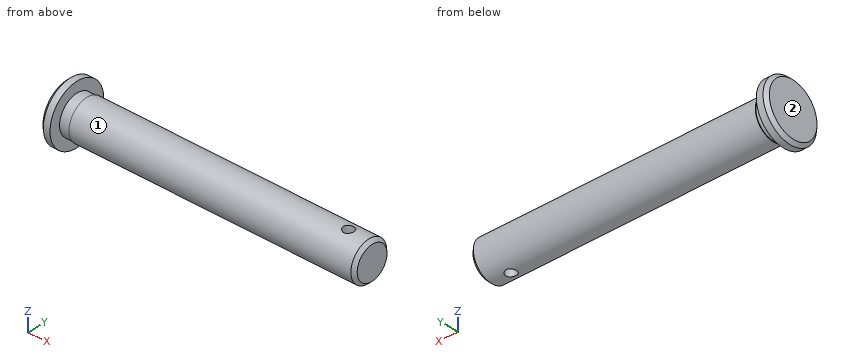
```python
from build123d import *

# Parameters (mm, degrees)
SKETCH2_R          = 0.8
CUT_EXTRUDE1_DEPTH = 46.15517689
CHAMFER1_SIZE      = 0.5


with BuildPart() as part:
    # Sketch1 → Revolve1 (revolve)
    with BuildSketch(Plane.XY, mode=Mode.PRIVATE) as revolve1_sk:
        Polygon((-1.5, 0), (-1.5, 4.5), (0, 4.5), (0, 2.9), (1.5, 2.9), (1.5, 3), (44.3, 3), (44.3, 0), align=None)
    revolve(revolve1_sk.sketch.rotate(Axis((0, 0, 0), (1, 0, 0)), 90), axis=Axis((0, 0, 0), (1, 0, 0)))

    # Sketch2 → Cut-Extrude1 (cut, through all)
    with BuildSketch(Plane.XY.offset(3)):
        with Locations((40.8, 0)):
            Circle(SKETCH2_R)
    extrude(amount=-CUT_EXTRUDE1_DEPTH, mode=Mode.SUBTRACT)

    # Chamfer1
    chamfer1_edges = [part.edges().sort_by_distance(p)[0] for p in [
        (44.3, 0, -3),
        (-1.5, 0, -4.5),
    ]]
    chamfer(chamfer1_edges, length=CHAMFER1_SIZE)


solid = part.part
```
Build history of the part. All positions in model axes, mm. Face numbers are marked on the shaded views. A direction names the side the tool comes from. Give positions to 0.01 mm unless a question says otherwise; leave off trailing zeros. Loops run counter-clockwise (first coordinate to the right, second up) from the corner with the lowest first, then second, coordinate; pieces in that order, holes last. Notation, with made-up numbers: (9, 51) - (24, 51) arc R11 cw to (24, 63) - close; hole circle Ø4 at (-10.5, 75). An arc over 180 degrees is marked (long way). Use a Markdown table: item, result.
(1) Which spindle directions (+Z, -Z, +X, -X, +Y, -Y) get a long thin tool onto all of the face, cutting with end or side? Do the marked faces 1 and 2. Say none if no direction does.
Taken from the geometry:
| item | result |
|---|---|
| face 1 | +X |
| face 2 | +Z, -Z, -X, +Y, -Y |
(2) Band-saw the part on A-A (y = 0). Give the cut face in (x, z), and give its area (3 significant figures).
Taken from the geometry:
| item | result |
|---|---|
| outline | (-1.5, -4) - (-1, -4.5) - (0, -4.5) - (0, -2.9) - (1.5, -2.9) - (1.5, -3) - (40, -3) - (40, 3) - (1.5, 3) - (1.5, 2.9) - (0, 2.9) - (0, 4.5) - (-1, 4.5) - (-1.5, 4) - close; (41.6, -3) - (43.8, -3) - (44.3, -2.5) - (44.3, 2.5) - (43.8, 3) - (41.6, 3) - close |
| area | 269 mm2 |
(3) Band-saw the part on B-B (x = 10). Give the cut face in (y, z).
Taken from the geometry:
| item | result |
|---|---|
| outline | circle Ø6 at (0, 0) |
(4) Wall check: line 1 along X through (y, z) = (0, 0.75); line 2 along Y through (x, z) = (40.8, 0); line 3 along X through (y, z) = (1, -3.5). Give the ranges that are in metal, low to high.
Taken from the geometry:
| item | result |
|---|---|
| line 1 | -1.5 to 40, 41.6 to 44.3 |
| line 2 | -3 to -0.8, 0.8 to 3 |
| line 3 | -1.5 to 0 |
(5) Band-saw the part on C-C (x = 40.8). Give the cut face in (y, z), and give its area (3 significant figures).
Taken from the geometry:
| item | result |
|---|---|
| outline | (-0.8, -2.89) - (-0.8, 2.89) arc R3 ccw to start; (0.8, -2.89) arc R3 ccw to (0.8, 2.89) - close |
| area | 18.8 mm2 |
(6) Drop flat-ended pins along their axis: pin 1 Ø2 at (x, y) = (23.5, -2.5) entering from +Z; pin 2 Ø1.5 at (x, z) = (3.5, 3.5) entering from -Y; pin 3 Ø3 at (x, z) = (35, 1) entering from +Y. Give the stop position or say it passes through.
Taken from the geometry:
| item | result |
|---|---|
| pin 1 | z = 2.6 |
| pin 2 | y = -1.2 |
| pin 3 | y = 3 |
